from build123d import *

# Parameters (mm, degrees)
F0_R     = 63.5
F1_DEPTH = 127


with BuildPart() as f1:
    # F0 (on Right) → F1 (new body)
    with BuildSketch(Plane.YZ):
        with BuildLine():
            Line((790.493007, 126.598885), (-435.038035, 126.417593))
            Line((-435.038035, 126.417593), (-459.372944, 126.413993))
            ThreePointArc((-459.372944, 126.413993), (-573.96915, -7.43188), (-444.519662, -126.971991))
            Line((-444.519662, -126.971991), (793.259037, -126.788887))
            Line((793.259037, -126.788887), (807.935979, -126.786715))
            ThreePointArc((807.935979, -126.786715), (927.571591, -1.348702), (810.627042, 126.601864))
            Line((810.627042, 126.601864), (790.493007, 126.598885))
        make_face()
        with Locations((-447.186789, 0)):
            Circle(F0_R, mode=Mode.SUBTRACT)
        with Locations((800.578752, 0)):
            Circle(F0_R, mode=Mode.SUBTRACT)
    extrude(amount=F1_DEPTH)


solid = f1.part
The model under review builds one solid part; all positions refer to its coordinate system, in mm. Give positions to 0.01 mm unless a question says otherwise; leave off trailing zeros. Loops run counter-clockwise (first coordinate to the right, second up) from the corner with the lowest first, then second, coordinate; pieces in that order, holes last. Notation, with made-up numbers: (7.5, 46) -> (28.5, 46) arc R20 cw to (28.5, 72) -> close; hole circle Ø9 at (24.25, 84). An arc over 180 degrees is marked (long way). Put each result on its own line as item: value. Start each with the question number.
1. We need section A-A on z = 0. State the section outline as (x, y) points.
2. We need section B-B on y = -415. State the section outline as (x, z) points, then the cut area to 3 significant figures.
3. We need section D-D on z = 105. State the section outline as (x, y) points.
4. We need section C-C on x = 93.5. State the section outline as (y, z) points, then the cut area to 3 significant figures.
5. Clearance check with flat-ended pins moving along their axes: P1, Ø1.5, axis at x = 94.5, z = 69, coming from the -Y side; P2, Ø5, axis at x = 82, z = 36, coming from the +Y side; P3, Ø1.5, axis at x = 51.5, y = -372, coming from the -Z side. State where each tip first meets the part, or that it passes through.
6. Wall thickness on probe 1 along Y at (x, z) = (47, -5.5); probe 2 along Y at (x, z) = (42, 15); probe 3 along Z at (x, y) = (28.5, -187): over which ranges is each line inside the solid? List them lowest first.
Determined:
1. outline: (0, -574.19) -> (127, -574.19) -> (127, -510.69) -> (0, -510.69) -> close; (0, -383.69) -> (127, -383.69) -> (127, 737.08) -> (0, 737.08) -> close; (0, 864.08) -> (127, 864.08) -> (127, 927.58) -> (0, 927.58) -> close
2. outline: (0, -126.97) -> (127, -126.97) -> (127, -54.74) -> (0, -54.74) -> close; (0, 54.74) -> (127, 54.74) -> (127, 126.42) -> (0, 126.42) -> close
2. area: 18,300 mm^2
3. outline: (0, -518.63) -> (127, -518.63) -> (127, 872.02) -> (0, 872.02) -> close
4. outline: (-459.37, 126.41) arc R127 ccw to (-444.52, -126.97) -> (807.94, -126.79) arc R127 ccw to (810.63, 126.6) -> close; hole circle Ø127 at (-447.19, 0); hole circle Ø127 at (800.58, 0)
4. area: 341,000 mm^2
5. P1: y = -554.29
5. P2: y = 923.08
5. P3: z = -126.96
6. probe 1: -574.07 to -510.45, -383.93 to 737.32, 863.84 to 927.46
6. probe 2: -573.3 to -508.89, -385.48 to 738.88, 862.28 to 926.69
6. probe 3: -126.93 to 126.45
